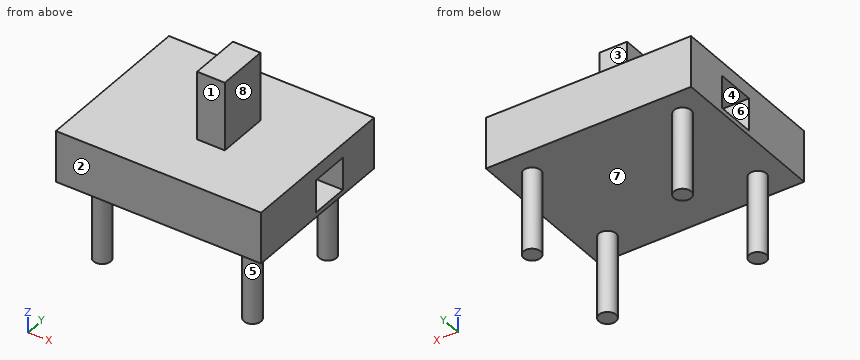
from build123d import *

# Parameters (mm, degrees)
F0_W     = 1524
F0_H     = 1219.2
F1_DEPTH = 381
F2_R     = 63.5
F3_DEPTH = 609.6
F4_W     = 288.1702780724
F4_H     = 241.9668510556
F5_DEPTH = 1524
F7_W     = 205.6101411581
F7_H     = 385.203063488
F8_DEPTH = 508


with BuildPart() as f1:
    # F0 (on Top) → F1 (new body)
    with BuildSketch(Plane.XY):
        Rectangle(F0_W, F0_H)
    extrude(amount=F1_DEPTH)

    # F2 (on face) → F3 (join)
    with BuildSketch(Plane(origin=(0, 0, 0), x_dir=(1, 0, 0), z_dir=(0, 0, -1))):
        with Locations((-558.8, -406.4)):
            Circle(F2_R)
        with Locations((-558.8, 406.4)):
            Circle(F2_R)
        with Locations((558.8, 406.4)):
            Circle(F2_R)
        with Locations((558.8, -406.4)):
            Circle(F2_R)
    extrude(amount=F3_DEPTH)

    # F4 (on face) → F5 (cut, through all)
    with BuildSketch(Plane.YZ.offset(762)):
        with Locations((129.0563344955, 157.3744080961)):
            Rectangle(F4_W, F4_H)
    extrude(amount=-F5_DEPTH, mode=Mode.SUBTRACT)

    # F7 (on face) → F8 (join)
    with BuildSketch(Plane.XY.offset(381)):
        with Locations((102.8050705791, 0)):
            Rectangle(F7_W, F7_H)
    extrude(amount=F8_DEPTH)


solid = f1.part
Design review of the part built by this model. Coordinates are the model's own, in mm. Face numbers are marked on the shaded views. A direction names the side the tool comes from. Round coordinates to 2 decimals unless told otherwise and drop trailing zeros. Write each loop counter-clockwise with the first axis right and the second up, starting at its lowest first coordinate (ties: lowest second). Pieces come first, ordered by that corner, then holes.
Item 1: Consider section A-A on z = 174. Give the boundary of the cut face in (x, y), and give its area (3 significant figures).
Item 2: Consider section C-C on x = 294. Give the boundary of the cut face in (y, z), and give its area (3 significant figures).
Item 3: Consider section D-D on y = 406.4. Give the boundary of the cut face in (x, z), and give its area (3 significant figures).
Item 4: Consider section B-B on y = 69. Give the boundary of the cut face in (x, z), and give its area (3 significant figures).
Item 5: For the marked faces 1, 2, 3, 4 and 5, list the 3-axis set-ups (+Z, -Z, +X, -X, +Y, -Y) from which the entire face can be reached by the end or side of a thin tool; tool diameter is ignored.
Item 6: Draft analysis for pull direction Z (two halves, no side actions). For the marked faces 6, 7 and 8, state which applies: released by +Z, released by -Z, zero draft, split by the parting line, or undercut.
Item 7: Wall thickness on L1, parallel to Z at x = 496.5, y = 102; L2, parallel to Y at x = -596.5, z = 129; L3, parallel to Z at x = 643.5, y = -92: over which ranges is each line inside the solid? List them lowest first.
Item 8: For pin 1 Ø1.5 at (x, y) = (-518, -428.5) entering from +Z; pin 2 Ø1.5 at (y, z) = (-152.5, 436.5) entering from -X; pin 3 Ø8 at (x, y) = (64, 149) entering from -Z, all flat-tipped, find the tip position at first contact; note any pin that passes through.
Check values:
1. outline: (-762, -609.6) - (762, -609.6) - (762, -15.03) - (-762, -15.03) - close; (-762, 273.14) - (762, 273.14) - (762, 609.6) - (-762, 609.6) - close
1. area: 1,420,000 mm2
2. outline: (-609.6, 0) - (609.6, 0) - (609.6, 381) - (-609.6, 381) - close; hole (-15.03, 36.39) - (273.14, 36.39) - (273.14, 278.36) - (-15.03, 278.36) - close
2. area: 395,000 mm2
3. outline: (-762, 0) - (-622.3, 0) - (-622.3, -609.6) - (-495.3, -609.6) - (-495.3, 0) - (495.3, 0) - (495.3, -609.6) - (622.3, -609.6) - (622.3, 0) - (762, 0) - (762, 381) - (-762, 381) - close
3. area: 735,000 mm2
4. outline: (-762, 0) - (762, 0) - (762, 36.39) - (-762, 36.39) - close; (-762, 278.36) - (762, 278.36) - (762, 381) - (205.61, 381) - (205.61, 889) - (0, 889) - (0, 381) - (-762, 381) - close
4. area: 316,000 mm2
5. face 1: +Z, +X, -X, -Y
5. face 2: +Z, -Z, +X, -X, -Y
5. face 3: +Z, +X, -X, +Y
5. face 4: +X, -X
5. face 5: -Z
6. face 6: undercut
6. face 7: released by -Z
6. face 8: zero draft
7. L1: z = 0 to 36.39, 278.36 to 381
7. L2: y = -609.6 to -15.03, 273.14 to 609.6
7. L3: z = 0 to 381
8. pin 1: stops at z = 381
8. pin 2: stops at x = 0
8. pin 3: stops at z = 0
